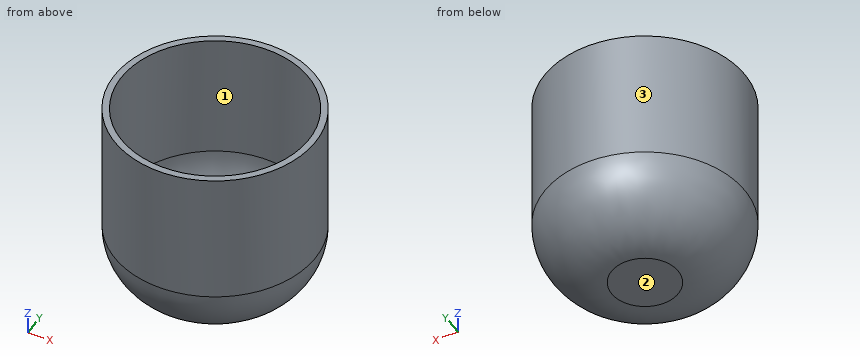
```python
from build123d import *

# Parameters (mm, degrees)
F0_R     = 42.0600289117
F1_DEPTH = 76.2
F2_T     = -2.54
F3_R     = 25.4
F4_R     = 39.5200289117
F5_DEPTH = 25.4
F8_R     = 38.1
F9_DEPTH = 76.2
F10_T    = -2.54
F11_R    = 25.4


with BuildPart() as f1:
    # F0 (on Top) → F1 (new body)
    with BuildSketch(Plane.XY):
        Circle(F0_R)
    extrude(amount=F1_DEPTH)

    # F2
    f2_openings = [f1.faces().sort_by_distance(p)[0] for p in [
        (0, 0, 76.2),
    ]]
    offset(amount=F2_T, openings=f2_openings)

    # F3
    f3_edges = [f1.edges().sort_by_distance(p)[0] for p in [
        (-39.520029, 0, 2.54),
        (-42.060029, 0, 0),
    ]]
    fillet(f3_edges, radius=F3_R)


with BuildPart() as f5:
    # F4 (on face) → F5 (new body)
    with BuildSketch(Plane.XY.offset(76.2)):
        Circle(F4_R)
    extrude(amount=F5_DEPTH)


with BuildPart() as f9:
    # F8 (on Top) → F9 (new body)
    with BuildSketch(Plane.XY):
        Circle(F8_R)
    extrude(amount=F9_DEPTH)

    # F10
    f10_openings = [f9.faces().sort_by_distance(p)[0] for p in [
        (0, 0, 76.2),
    ]]
    offset(amount=F10_T, openings=f10_openings)

    # F11
    f11_edges = [f9.edges().sort_by_distance(p)[0] for p in [
        (-35.56, 0, 2.54),
        (-38.1, 0, 0),
    ]]
    fillet(f11_edges, radius=F11_R)


solid = f9.part
```
Here's how the part is built. I have some questions about the finished solid (model axes, mm). Face numbers are marked on the shaded views. Coordinates: 2 decimals unless noted, no trailing zeros. Write each loop counter-clockwise with the first axis right and the second up, starting at its lowest first coordinate (ties: lowest second). Pieces come first, ordered by that corner, then holes. Notation, with made-up numbers: (-6.5, -40) -> (8.5, -40) arc R34 cw to (8.5, -6) -> close; hole circle Ø5 at (78.25, 23). An arc over 180 degrees is marked (long way). Use a Markdown table: item, result. Add a question column.
(1) I'm going to push flat-ended pins straight in: P1, Ø16.5, axis at x = 0, y = 4.5, coming from the +Z side; P2, Ø8, axis at x = 2, y = 19, coming from the +Z side; P3, Ø12, axis at x = 25.5, y = 2.5, coming from the -Z side. Where does each tip first touch, or does it pass through?
(2) Please list where these lines run through material, in increasing order: line 1 (Y direction, x = 0, z = 47); line 2 (X direction, y = 18, z = 28.5); line 3 (Y direction, x = -6.5, z = 36).
(3) We'd pull the mould along X, two halves only. Please class the marked faces 1, 2 and 3: +X half, -X half, draft (parallel to the pull), parting line (faces both ways), or undercut.
(4) If we section it at A-A, the plane z = 39: Write out the boundary of the cut face in (x, y).
Outcome:
| question | item | result |
|---|---|---|
| 1 | P1 | stops at z = 2.67 |
| 1 | P2 | stops at z = 6.09 |
| 1 | P3 | stops at z = 0.96 |
| 2 | line 1 | y = -38.1 to -35.56, 35.56 to 38.1 |
| 2 | line 2 | x = -33.58 to -30.67, 30.67 to 33.58 |
| 2 | line 3 | y = -37.54 to -34.96, 34.96 to 37.54 |
| 3 | face 1 | undercut |
| 3 | face 2 | draft |
| 3 | face 3 | parting line |
| 4 | outline | circle Ø76.2 at (0, 0); hole circle Ø71.12 at (0, 0) |
